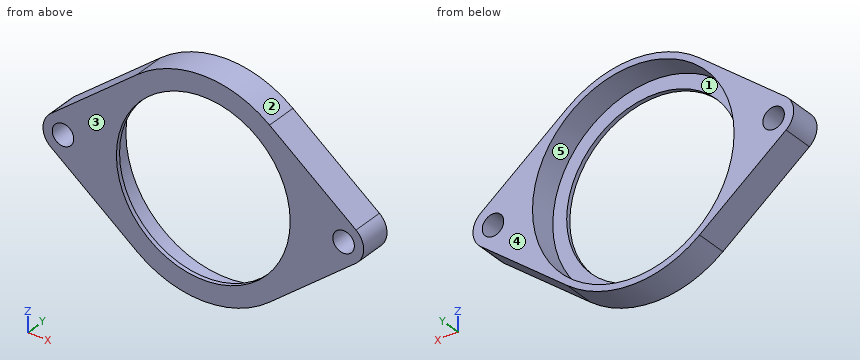
Autodesk Inventor part; units mm, degrees
ref_plane "YZ Plane" through (0, 0, 0) normal (1, 0, 0) x (0, 1, 0)
ref_plane "XZ Plane" through (0, 0, 0) normal (0, 1, 0) x (-1, 0, 0)
ref_plane "XY Plane" through (0, 0, 0) normal (0, 0, 1) x (1, 0, 0)
sketch "Sketch1" plane through (0, 0, 0) normal (0, 1, 0) x (-1, 0, 0)
  circle A0 centre (0, 0) radius 23.8125 construction
  line L0 (33.3248, 0) -> (-33.3248, 0) construction
  circle A1 centre (33.3248, 0) radius 4.7625 construction
  circle A2 centre (-33.3248, 0) radius 4.7625 construction
  circle A3 centre (0, 0) radius 20.6375
  circle A4 centre (0, 0) radius 25.4 construction
  line L1 (36.2741, 3.7394) -> (15.7298, 19.9433)
  line L2 (36.2741, -3.7394) -> (15.7298, -19.9433)
  line L3 (-15.7298, -19.9433) -> (-36.2741, -3.7394)
  line L4 (-36.2741, 3.7394) -> (-15.7298, 19.9433)
  arc A5 (15.7298, 19.9433) -> (-15.7298, 19.9433) centre (0, 0) ccw
  arc A6 (-15.7298, -19.9433) -> (15.7298, -19.9433) centre (0, 0) ccw
  arc A7 (36.2741, -3.7394) -> (36.2741, 3.7394) centre (33.3248, 0) ccw
  arc A8 (-36.2741, 3.7394) -> (-36.2741, -3.7394) centre (-33.3248, 0) ccw
  point P0 (-36.2741, -3.7394)
  dimension "d0" = 47.625
  dimension "d1" = 33.3248
  dimension "d2" = 9.525
  dimension "d3" = 3.175
  dimension "d4" = 1.5875
extrude "Extrusion1" add sketch "Sketch1" along normal blind 7.62
sketch "Sketch2" plane through (0, 7.62, 0) normal (0, 1, 0) x (1, 0, 0)
  circle A0 centre (0, 0) radius 23.9395
  dimension "d7" = 47.879
extrude "Extrusion2" cut sketch "Sketch2" against normal blind 6.604
hole "Hole1" at (-33.3248, 0, 0) at (33.3248, 0, 0) direction (0, 1, 0) diameter 5.1054 end through all
properties part number "EL2-CGB-008" material "Aluminum 6061"
Read the model definition and answer for the solid it produces. Units are mm, in the model's axes. Face numbers are marked on the shaded views. A direction names the side the tool comes from. Round coordinates to 2 decimals unless told otherwise and drop trailing zeros. Write each loop counter-clockwise with the first axis right and the second up, starting at its lowest first coordinate (ties: lowest second). Pieces come first, ordered by that corner, then holes.
1. Given pin 1 Ø2 at (y, z) = (1, -19.5) entering from -X; pin 2 Ø1 at (x, z) = (-19, -16.5) entering from -Y; pin 3 Ø1 at (y, z) = (6, -3.5) entering from +X; pin 4 Ø4 at (x, y) = (28, 2.5) entering from +Z, each flat-ended and moving along its own axis, determine where each tip first touches the part or whether it passes through.
2. The part is cut by section A-A, the plane x = 0. Determine the outline of the cut face in (y, z).
3. The part is cut by section B-B, the plane z = 18.5. Determine the outline of the cut face in (x, y), then the cut area to 3 significant figures.
4. The part is cut by section C-C, the plane z = 0. Determine the outline of the cut face in (x, y).
5. Straight lines are drawn through the part: L1, parallel to X at y = 1.75, z = 0; L2, parallel to X at y = 0.55, z = 0; L3, parallel to Z at x = -0.5, y = 0.75. For each, find the intervals that lie inside material, in ascending order.
6. Which of the six approach directions +Z, -Z, +X, -X, +Y, -Y give full straight-line access (tool end or side, diameter ignored) to the marked faces 4 and 5?
7. The part is cut by section D-D, the plane y = 5.75. Determine the outline of the cut face in (x, z).
8. Determine the mould class of the marked faces 1, 2 and 3 for opening direction X: pulls with the +X half, pulls with the -X half, needs draft (parallel to the pull), parting line crosses it, or undercut.
Values:
1. pin 1: stops at x = -17.56
1. pin 2: stops at y = 0
1. pin 3: stops at x = 37.02
1. pin 4: stops at z = 11.84
2. outline: (0, -25.4) - (7.62, -25.4) - (7.62, -23.94) - (1.02, -23.94) - (1.02, -20.64) - (0, -20.64) - close; (0, 20.64) - (1.02, 20.64) - (1.02, 23.94) - (7.62, 23.94) - (7.62, 25.4) - (0, 25.4) - close
3. outline: (-17.56, 0) - (-9.15, 0) - (-9.15, 1.02) - (-15.19, 1.02) - (-15.19, 7.62) - (-17.56, 7.62) - close; (9.15, 0) - (17.56, 0) - (17.56, 7.62) - (15.19, 7.62) - (15.19, 1.02) - (9.15, 1.02) - close
3. area: 48.3 mm2
4. outline: (-38.09, 0) - (-35.88, 0) - (-35.88, 7.62) - (-38.09, 7.62) - close; (-30.77, 0) - (-20.64, 0) - (-20.64, 1.02) - (-23.94, 1.02) - (-23.94, 7.62) - (-30.77, 7.62) - close; (20.64, 0) - (30.77, 0) - (30.77, 7.62) - (23.94, 7.62) - (23.94, 1.02) - (20.64, 1.02) - close; (35.88, 0) - (38.09, 0) - (38.09, 7.62) - (35.88, 7.62) - close
5. L1: x = -38.09 to -35.88, -30.77 to -23.94, 23.94 to 30.77, 35.88 to 38.09
5. L2: x = -38.09 to -35.88, -30.77 to -20.64, 20.64 to 30.77, 35.88 to 38.09
5. L3: z = -25.4 to -20.63, 20.63 to 25.4
6. face 4: +Z, -Z, +X, -X, +Y
6. face 5: +Y
7. outline: (-36.27, -3.74) - (-15.73, -19.94) arc R25.4 ccw to (15.73, -19.94) - (36.27, -3.74) arc R4.76 ccw to (36.27, 3.74) - (15.73, 19.94) arc R25.4 ccw to (-15.73, 19.94) - (-36.27, 3.74) arc R4.76 ccw to start; hole circle Ø5.11 at (-33.32, 0); hole circle Ø47.88 at (0, 0); hole circle Ø5.11 at (33.32, 0)
8. face 1: undercut
8. face 2: parting line crosses it
8. face 3: needs draft
